from build123d import *

# Parameters (mm, degrees)
SKETCH2_W           = 292.1
SKETCH2_H           = 203.2
BOSS_EXTRUDE1_DEPTH = 12.7
SKETCH3_W           = 292.1
SKETCH3_H           = 203.2
SKETCH3_W_2         = 266.7
SKETCH3_H_2         = 177.8
BOSS_EXTRUDE2_DEPTH = 88.9
CUT_EXTRUDE1_REACH  = 368.764
SKETCH4_W           = 152.4
SKETCH4_H           = 63.5


with BuildPart() as part:
    # Sketch2 → Boss-Extrude1 (new body)
    with BuildSketch(Plane(origin=(0, 0, 0), x_dir=(1, 0, 0), z_dir=(0, 1, 0))):
        with Locations((146.05, 101.6)):
            Rectangle(SKETCH2_W, SKETCH2_H)
    extrude(amount=BOSS_EXTRUDE1_DEPTH)

    # Sketch3 → Boss-Extrude2 (add)
    with BuildSketch(Plane.XZ):
        with Locations((146.05, -101.6)):
            Rectangle(SKETCH3_W, SKETCH3_H)
        with Locations((146.05, -101.6)):
            Rectangle(SKETCH3_W_2, SKETCH3_H_2, mode=Mode.SUBTRACT)
    extrude(amount=BOSS_EXTRUDE2_DEPTH)

    # Sketch4 → Cut-Extrude1 (cut, up to next)
    with BuildSketch(Plane.ZY, mode=Mode.PRIVATE) as cut_extrude1_sk1:
        with Locations((-101.6, -57.15)):
            Rectangle(SKETCH4_W, SKETCH4_H)
    cut_extrude1_tool1 = extrude(cut_extrude1_sk1.sketch, amount=-CUT_EXTRUDE1_REACH, mode=Mode.PRIVATE) & part.part
    add(cut_extrude1_tool1.solids().sort_by_distance((0, -57.15, -101.6))[0], mode=Mode.SUBTRACT)


solid = part.part
Part model, mm, in its own coordinate system. A direction names the side the tool comes from. Coordinates: 2 decimals unless noted, no trailing zeros. Order: outer loops, then holes, each group sorted by start corner. A loop starts at its lowest first (then second) coordinate and runs counter-clockwise, first axis right, second up.
(1) Slice it at B-B, the plane z = -17.5. Write the cut outline in (x, y), and give its area (3 significant figures).
Check sheet entries:
outline: (0, -88.9) - (12.7, -88.9) - (12.7, 0) - (279.4, 0) - (279.4, -88.9) - (292.1, -88.9) - (292.1, 12.7) - (0, 12.7) - close
area: 5,970 mm2
(2) Pin check, flat tips, straight feed: pin 1 Ø8 at (x, y) = (29.5, -4.5) entering from +Z; pin 2 Ø5 at (x, z) = (122.5, -111) entering from -Y; pin 3 Ø6.5 at (x, z) = (3, -70) entering from -Y. Stop position of each tip, or through.
Check sheet entries:
pin 1: stops at z = 0
pin 2: stops at y = 0
pin 3: stops at y = -25.4
(3) Probe L1, parallel to Z at x = 186, y = -27; L2, parallel to X at y = -49, z = -185.5; L3, parallel to X at y = -39, z = -168.5. List the from-to ranges inside material, lowest first.
Check sheet entries:
L1: z = -203.2 to -190.5, -12.7 to 0
L2: x = 0 to 12.7, 279.4 to 292.1
L3: x = 279.4 to 292.1
(4) Slice it at C-C, the plane y = -39.5. Write the cut outline in (x, z), and give its area (4 significant figures).
Check sheet entries:
outline: (0, -203.2) - (292.1, -203.2) - (292.1, 0) - (0, 0) - (0, -25.4) - (12.7, -25.4) - (12.7, -12.7) - (279.4, -12.7) - (279.4, -190.5) - (12.7, -190.5) - (12.7, -177.8) - (0, -177.8) - close
area: 10,000 mm2
(5) Tool access for faces 1 (the face through (0, -15, -103)), 2 (the face through (12.7, -24, -103)), 3 (the face through (6, -25.4, -103)): list every direction of +Z, -Z, +X, -X, +Y, -Y with a clear straight run to the whole face (end or side of a thin tool).
Check sheet entries:
face 1: +Z, -Z, -X, +Y, -Y
face 2: -Y
face 3: -X, -Y
(6) Pull direction Z, two halves, no side cores. Call faces 4 (the face through (167, -88.9, -191)), 5 (the face through (144, -37, 0)), 6 (the face through (6, -58, -177.8)): pulls with the +Z half, pulls with the -Z half, needs draft (parallel to the pull), parting line crosses it, or undercut.
Check sheet entries:
face 4: needs draft
face 5: pulls with the +Z half
face 6: undercut
(7) Slice it at A-A, the plane x = 268.5. Write the cut outline in (y, z), and give its area (3 significant figures).
Check sheet entries:
outline: (-88.9, -203.2) - (12.7, -203.2) - (12.7, 0) - (-88.9, 0) - (-88.9, -12.7) - (0, -12.7) - (0, -190.5) - (-88.9, -190.5) - close
area: 4,840 mm2
